The model under review builds one solid part; all positions refer to its coordinate system, in mm. Face numbers are marked on the shaded views. A direction names the side the tool comes from. Give positions to 0.01 mm unless a question says otherwise; leave off trailing zeros. Loops run counter-clockwise (first coordinate to the right, second up) from the corner with the lowest first, then second, coordinate; pieces in that order, holes last. Notation, with made-up numbers: M 26.5,45 L 43.5,45 A6 cw 43.5,53 Z; hole C 73,-20.75 d11. An arc over 180 degrees is marked long. Write item = value, one per line. Start each with the question number.
1. For the marked faces 5 and 6, list the 3-axis set-ups (+Z, -Z, +X, -X, +Y, -Y) from which the entire face can be reached by the end or side of a thin tool; tool diameter is ignored.
2. We need section A-A on x = -110. Give the boundary of the cut face in (y, z).
3. We need section D-D on y = -289.5. Give the boundary of the cut face in (x, z), then the cut area to 3 significant figures.
4. Wall thickness on line 1 along Z through (x, y) = (-106.5, -269); line 2 along Y through (x, z) = (-89, 13.5); line 3 along X through (y, z) = (-278.5, 31): over which ranges is each line inside the solid? List them lowest first. Write a range as from..to.
5. We need section B-B on y = -267. Give the boundary of the cut face in (x, z), then the cut area to 3 significant figures.
6. Draft analysis for pull direction Z (two halves, no side actions). For the marked faces 1, 2, 3 and 4, state which applies: pulls with the +Z half, pulls with the -Z half, needs draft (parallel to the pull), parting line crosses it, or undercut.
7. For pin 1 (8 mm diameter, centred on x = -85.5, z = 66, fed in from +Y); pin 2 (1 mm diameter, centred on x = -89, z = 75.5, fed in from -Y); pin 3 (8 mm diameter, centred on x = -99.5, z = 72, fed in from +Y); pin 4 (4 mm diameter, centred on y = -300, z = 39.5, fed in from -X) (3 decimals), all flat-tipped, find the tip position at first contact; note any pin that passes through.
8. We need section C-C on x = -84. Give the boundary of the cut face in (y, z).
from build123d import *

# Parameters (mm, degrees)
SKETCH1_W           = 42.467218632
SKETCH1_H           = 42.674431579
BOSS_EXTRUDE1_DEPTH = 10
SKETCH2_R           = 12.637375282
BOSS_EXTRUDE2_DEPTH = 89
SKETCH4_W           = 42.467218632
SKETCH4_H           = 42.674431579
BOSS_EXTRUDE3_DEPTH = 10
FILLET1_R           = 2


with BuildPart() as part:
    # Sketch1 → Boss-Extrude1 (new body)
    with BuildSketch(Plane.XY):
        with Locations((-94.578448042, -284.38200622)):
            Rectangle(SKETCH1_W, SKETCH1_H)
    extrude(amount=BOSS_EXTRUDE1_DEPTH)

    # Sketch2 → Boss-Extrude2 (add)
    with BuildSketch(Plane.XY.offset(10)):
        with Locations((-94.578448042, -284.38200622)):
            Circle(SKETCH2_R)
    extrude(amount=BOSS_EXTRUDE2_DEPTH)

    # Sketch4 → Boss-Extrude3 (add)
    with BuildSketch(Plane(origin=(0, 0, 105), x_dir=(-1, 0, 0), z_dir=(0, 0, -1))):
        with Locations((94.578448042, -284.38200622)):
            Rectangle(SKETCH4_W, SKETCH4_H)
    extrude(amount=BOSS_EXTRUDE3_DEPTH)

    # Fillet1
    fillet1_edges = [part.edges().sort_by_distance(p)[0] for p in [
        (-73.344838726, -263.044790431, 100),
        (-73.344838726, -305.71922201, 100),
        (-115.812057358, -305.71922201, 100),
        (-115.812057358, -263.044790431, 100),
        (-73.344838726, -305.71922201, 5),
        (-115.812057358, -305.71922201, 5),
        (-115.812057358, -263.044790431, 5),
        (-73.344838726, -263.044790431, 5),
    ]]
    fillet(fillet1_edges, radius=FILLET1_R)


solid = part.part
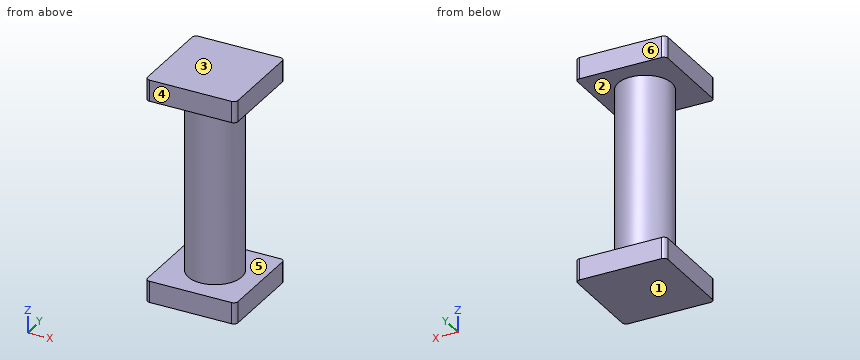
Final values:
q1.face_5 = none
q1.face_6 = +Z, -Z, +X, -X, +Y
q2.outline = M -305.72,0 L -263.04,0 L -263.04,10 L -305.72,10 Z; M -305.72,95 L -263.04,95 L -263.04,105 L -305.72,105 Z
q3.outline = M -115.81,0 L -73.34,0 L -73.34,10 L -83.02,10 L -83.02,95 L -73.34,95 L -73.34,105 L -115.81,105 L -115.81,95 L -106.13,95 L -106.13,10 L -115.81,10 Z
q3.area = 2,810 mm²
q4.line_1 = 0..10, 95..105
q4.line_2 = -295.72..-273.04
q4.line_3 = -105.76..-83.39
q5.outline = M -115.81,0 L -73.34,0 L -73.34,10 L -115.81,10 Z; M -115.81,95 L -73.34,95 L -73.34,105 L -115.81,105 Z
q5.area = 849 mm²
q6.face_1 = pulls with the -Z half
q6.face_2 = undercut
q6.face_3 = pulls with the +Z half
q6.face_4 = needs draft
q7.pin_1 = -272.81
q7.pin_2 = -295.95
q7.pin_3 = -271.78
q7.pin_4 = through
q8.outline = M -305.72,0 L -263.04,0 L -263.04,10 L -277.47,10 L -277.47,95 L -263.04,95 L -263.04,105 L -305.72,105 L -305.72,95 L -291.3,95 L -291.3,10 L -305.72,10 Z
